Build history of the part. All positions in model axes, mm. A direction names the side the tool comes from. Round coordinates to 2 decimals unless told otherwise and drop trailing zeros. Write each loop counter-clockwise with the first axis right and the second up, starting at its lowest first coordinate (ties: lowest second). Pieces come first, ordered by that corner, then holes.
Item 1: Wall check: probe 1 along Z at (x, y) = (7.5, 4.25) (3 decimals); probe 2 along Y at (x, z) = (3.75, 6.5); probe 3 along Y at (x, z) = (7.25, 1.75). Give the ranges that are in metal, low to high.
Item 2: Band-saw the part on A-A, the plane x = 4. Write the cut outline in (y, z) (3 decimals), then the cut area to 3 significant figures.
Item 3: Band-saw the part on B-B, the plane z = 7.25. Write the cut outline in (x, y).
Item 4: 3-axis set-ups, long thin cutter, end or side, ignore diameter. For faces 4 (the flat face through (4.45, 2.64, 8.81)), 5 (the flat face through (8, 12.141, 5)): which of +Z, -Z, +X, -X, +Y, -Y reach the whole face in a straight line?
Item 5: Band-saw the part on C-C, the plane y = 5. Write the cut outline in (x, z) (3 decimals), then the cut area to 3 significant figures.
Item 6: Band-saw the part on D-D, the plane y = 9.25. Write the cut outline in (x, z) (3 decimals), then the cut area to 3 significant figures.
Item 7: Mould opens along Z. For faces 1 (the flat face through (4.45, 9.52, 8.79)), 2 (the flat face through (0, 6, 5)), 3 (the flat face through (8, 6, 0)) say: +Z half, -Z half, draft (parallel to the pull), parting line (faces both ways), or undercut.
```python
from build123d import *

# Parameters (mm, degrees)
SKETCH1_W           = 16.4592
SKETCH1_H           = 12.1412
BOSS_EXTRUDE1_DEPTH = 10.795
SKETCH2_W           = 2.9972
SKETCH2_H           = 5.461
CUT_EXTRUDE1_DEPTH  = 9.017


with BuildPart() as part:
    # Sketch1 → Boss-Extrude1 (new body)
    with BuildSketch(Plane.XY):
        with Locations((8.2296, 6.0706)):
            Rectangle(SKETCH1_W, SKETCH1_H)
    extrude(amount=BOSS_EXTRUDE1_DEPTH)

    # Sketch2 → Cut-Extrude1 (cut)
    with BuildSketch(Plane.ZY):
        Polygon((1.524, 1.778), (1.524, 10.3632), (7.945751337, 10.3632), (9.652, 8.656951337), (9.652, 3.484248663), (7.945751337, 1.778), align=None)
        with Locations((5.4356, 6.0706)):
            Rectangle(SKETCH2_W, SKETCH2_H, mode=Mode.SUBTRACT)
    extrude(amount=-CUT_EXTRUDE1_DEPTH, mode=Mode.SUBTRACT)


solid = part.part
```
Results:
1. probe 1: z = 0 to 1.524, 3.937 to 6.934, 9.652 to 10.795
1. probe 2: y = 0 to 1.78, 3.34 to 8.8, 10.36 to 12.14
1. probe 3: y = 0 to 1.78, 10.36 to 12.14
2. outline: (0, 0) - (12.141, 0) - (12.141, 10.795) - (0, 10.795) - close; (3.34, 3.937) - (8.801, 3.937) - (8.801, 6.934) - (3.34, 6.934) - close; hole (1.778, 1.524) - (10.363, 1.524) - (10.363, 7.946) - (8.657, 9.652) - (3.484, 9.652) - (1.778, 7.946) - close
2. area: 80.6 mm2
3. outline: (0, 0) - (16.46, 0) - (16.46, 12.14) - (0, 12.14) - (0, 10.36) - (9.02, 10.36) - (9.02, 1.78) - (0, 1.78) - close
4. face 4: -X
4. face 5: +Z, -Z, +X, -X, +Y
5. outline: (0, 0) - (16.459, 0) - (16.459, 10.795) - (0, 10.795) - (0, 9.652) - (9.017, 9.652) - (9.017, 6.934) - (0, 6.934) - (0, 3.937) - (9.017, 3.937) - (9.017, 1.524) - (0, 1.524) - close
5. area: 131 mm2
6. outline: (0, 0) - (16.459, 0) - (16.459, 10.795) - (0, 10.795) - (0, 9.059) - (9.017, 9.059) - (9.017, 1.524) - (0, 1.524) - close
6. area: 110 mm2
7. face 1: undercut
7. face 2: draft
7. face 3: -Z half
